Design review of the part built by this model. Coordinates are the model's own, in mm. A direction names the side the tool comes from. Coordinates: 2 decimals unless noted, no trailing zeros. Loops run counter-clockwise (first coordinate to the right, second up) from the corner with the lowest first, then second, coordinate; pieces in that order, holes last.
Q1. Wall thickness on probe 1 along Y at (x, z) = (0, 0); probe 2 along Y at (x, z) = (0, 13.7); probe 3 along Y at (x, z) = (-7, 6): over which ranges is each line inside the solid? List them lowest first.
Q2. Machinability: for faces 1 (the face through (-6.94, -31.24, 0.21)), 2 (the face through (8, 67, 15)), 3 (the face through (-16.778, 43.292, 0.07)), 4 (the face through (-5.961, -26.846, 12.465)), 5 (the face through (8, 67, -15)), which of the approach directions +Z, -Z, +X, -X, +Y, -Y give a long, thin tool a straight path to every point of the face, cutting with its end or side? Answer none if there is none.
Q3. Add section A-A on z = 11.5. Give the boundary of the cut face in (x, y).
Q4. Add section B-B on y = 0. Give the boundary of the cut face in (x, z), and give its area (3 significant figures).
Q5. Draft analysis for pull direction X (two halves, no side actions). For faces 6 (the face through (0, 42, -5)), 7 (the face through (-2.47, 93.84, 0.21)), 8 (the face through (-2.799, 21.317, 19.86)), state which applies: released by +X, released by -X, zero draft, split by the parting line, or undercut.
Q6. Add section C-C on x = 0. Give the boundary of the cut face in (y, z), and give its area (4 significant figures).
Q7. For P1, Ø12, axis at x = 0, y = 75, coming from the +Z side; P2, Ø6, axis at y = 32.5, z = 6.5, coming from the +X side; P3, Ø3, axis at x = -3.5, z = 24.5, coming from the +Y side; P4, Ø2, axis at x = 12.5, z = 20, coming from the -Y side, all flat-tipped, find the tip position at first contact; note any pin that passes through.
Q8. Add section D-D on y = 75. Give the boundary of the cut face in (x, z).
```python
from build123d import *

# Parameters (mm, degrees)
BOSS_EXTRU_1_DEPTH      = 5
ESQUISSE1_3_R           = 19
ESQUISSE1_3_R_2         = 10
BOSS_EXTRU_2_DEPTH      = 15
ESQUISSE1_5_R           = 21.5
ESQUISSE1_5_R_2         = 17
BOSS_EXTRU_3_DEPTH      = 30
BOSS_EXTRU_3_DEPTH_BACK = 15
ESQUISSE1_6_R           = 32
ESQUISSE1_6_R_2         = 27.5
ESQUISSE1_6_R_3         = 21.5
BOSS_EXTRU_4_DEPTH      = 15
ENL_V_START             = 10
ESQUISSE1_7_R           = 27.5
ESQUISSE1_7_R_2         = 21.5
ENL_V_MAT_EXTRU_1_DEPTH = 5


with BuildPart() as part:
    # Esquisse1 → Boss.-Extru.1 (new body, symmetric)
    with BuildSketch(Plane.XY):
        with BuildLine():
            ThreePointArc((-26.678302647, 17.671111111), (0, 32), (26.678302647, 17.671111111))
            ThreePointArc((26.678302647, 17.671111111), (16.836772686, 42.914041255), (18.321243986, 69.966907631))
            ThreePointArc((18.321243986, 69.966907631), (0, 56), (-18.321243986, 69.966907631))
            ThreePointArc((-18.321243986, 69.966907631), (-16.836772686, 42.914041255), (-26.678302647, 17.671111111))
        make_face()
    extrude(amount=BOSS_EXTRU_1_DEPTH, both=True)

    # Esquisse1_3 → Boss.-Extru.2 (add, symmetric)
    with BuildSketch(Plane.XY):
        with Locations((0, 75)):
            Circle(ESQUISSE1_3_R)
        with Locations((0, 75)):
            Circle(ESQUISSE1_3_R_2, mode=Mode.SUBTRACT)
    extrude(amount=BOSS_EXTRU_2_DEPTH, both=True)



with BuildPart() as body_2:
    # Esquisse1_5 → Boss.-Extru.3 (new body, two sides)
    with BuildSketch(Plane.XY) as boss_extru_3_sk:
        Circle(ESQUISSE1_5_R)
        Circle(ESQUISSE1_5_R_2, mode=Mode.SUBTRACT)
    extrude(amount=BOSS_EXTRU_3_DEPTH)
    extrude(boss_extru_3_sk.sketch, amount=-BOSS_EXTRU_3_DEPTH_BACK)


with BuildPart() as part_1:
    add(part.part)

    add(body_2.part)  # Boss.-Extru.4 merges body 2
    # Esquisse1_6 → Boss.-Extru.4 (add, symmetric)
    with BuildSketch(Plane.XY):
        Circle(ESQUISSE1_6_R)
        Circle(ESQUISSE1_6_R_2, mode=Mode.SUBTRACT)
        Circle(ESQUISSE1_6_R_2)
        Circle(ESQUISSE1_6_R_3, mode=Mode.SUBTRACT)
    extrude(amount=BOSS_EXTRU_4_DEPTH, both=True)

    # Esquisse1_7 → Enl_v. mat.-Extru.1 (cut)
    with BuildSketch(Plane.XY.offset(ENL_V_START)):
        Circle(ESQUISSE1_7_R)
        Circle(ESQUISSE1_7_R_2, mode=Mode.SUBTRACT)
    extrude(amount=ENL_V_MAT_EXTRU_1_DEPTH, mode=Mode.SUBTRACT)


solid = part_1.part
```
Entries:
1. probe 1: y = -32 to -17, 17 to 65, 85 to 94
1. probe 2: y = -32 to -27.5, -21.5 to -17, 17 to 21.5, 27.5 to 32, 56 to 65, 85 to 94
1. probe 3: y = -31.22 to -15.49, 15.49 to 31.22, 57.34 to 67.86, 82.14 to 92.66
2. face 1: none
2. face 2: +Z, +X, -X, +Y
2. face 3: +Z, -Z, -X
2. face 4: +Z
2. face 5: -Z, +X, -X, +Y, -Y
3. outline: circle Ø64 at (0, 0); circle Ø43 at (0, 0); circle Ø38 at (0, 75); hole circle Ø55 at (0, 0); hole circle Ø34 at (0, 0); hole circle Ø20 at (0, 75)
4. outline: (-32, -15) - (-17, -15) - (-17, 30) - (-21.5, 30) - (-21.5, 10) - (-27.5, 10) - (-27.5, 15) - (-32, 15) - close; (17, -15) - (32, -15) - (32, 15) - (27.5, 15) - (27.5, 10) - (21.5, 10) - (21.5, 30) - (17, 30) - close
4. area: 975 mm2
5. face 6: zero draft
5. face 7: split by the parting line
5. face 8: undercut
6. outline: (-32, -15) - (-17, -15) - (-17, 30) - (-21.5, 30) - (-21.5, 10) - (-27.5, 10) - (-27.5, 15) - (-32, 15) - close; (17, -15) - (32, -15) - (32, -5) - (56, -5) - (56, -15) - (65, -15) - (65, 15) - (56, 15) - (56, 5) - (32, 5) - (32, 15) - (27.5, 15) - (27.5, 10) - (21.5, 10) - (21.5, 30) - (17, 30) - close; (85, -15) - (94, -15) - (94, 15) - (85, 15) - close
6. area: 1,755 mm2
7. P1: passes through
7. P2: stops at x = 20.35
7. P3: stops at y = 21.41
7. P4: stops at y = -18.17
8. outline: (-19, -15) - (-10, -15) - (-10, 15) - (-19, 15) - close; (10, -15) - (19, -15) - (19, 15) - (10, 15) - close
